The drawing under review shows one solid part. Ordinate dimensions are in mm from its lowest x, y, z. A direction names the side the tool comes from. Round coordinates to 2 decimals unless told otherwise and drop trailing zeros. Order: outer loops, then holes, each group sorted by start corner. A loop starts at its lowest first (then second) coordinate and runs counter-clockwise, first axis right, second up.
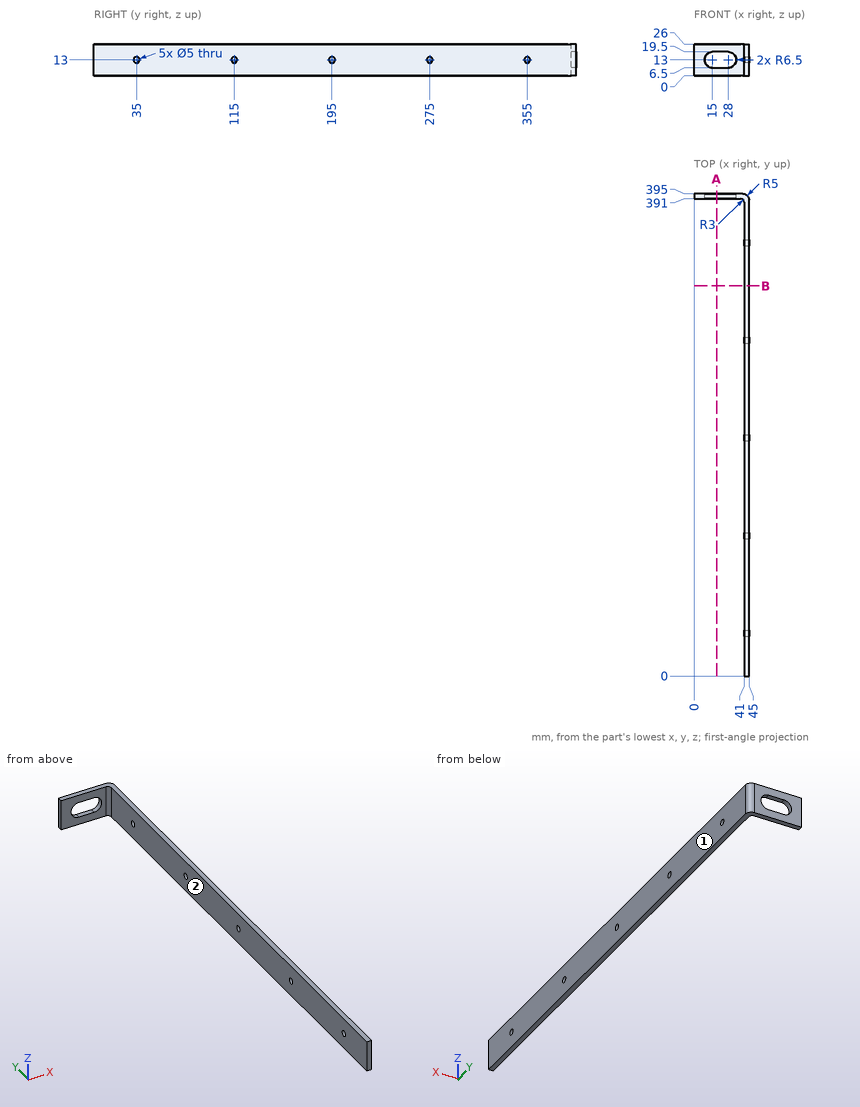
Q1. Clearance check with flat-ended pins moving along their axes: pin 1 (6.5 mm diameter, centred on y = 355, z = 13, fed in from -X); pin 2 (10 mm diameter, centred on x = 5.5, z = 19, fed in from -Y). State where each tip first meets the part, or that it passes through.
Q2. Take a section at A-A, the plane x = 18.5. State the section outline as (y, z) points, plus the area to 3 significant figures.
Q3. Wall thickness on line 1 (Z direction, x = 42.75, y = 195); line 2 (Y direction, x = 42.45, z = 13); line 3 (Y direction, x = 41.9, z = 13): over which ranges is each line inside the solid? List them lowest first.
Q4. Take a section at B-B, the plane y = 319.5. State the section outline as (x, z) points, plus the area to 3 significant figures.
Q5. Tool access review of the marked faces 1 and 2: name each direction out of +Z, -Z, +X, -X, +Y, -Y from which nothing blocks a thin tool from reaching the whole face with its end or side.
Working result:
1. pin 1: stops at x = 41
1. pin 2: stops at y = 391
2. outline: (391, 0) - (395, 0) - (395, 6.5) - (391, 6.5) - close; (391, 19.5) - (395, 19.5) - (395, 26) - (391, 26) - close
2. area: 52.0 mm2
3. line 1: z = 0 to 10.5, 15.5 to 26
3. line 2: y = 0 to 32.5, 37.5 to 112.5, 117.5 to 192.5, 197.5 to 272.5, 277.5 to 352.5, 357.5 to 394.36
3. line 3: y = 0 to 32.5, 37.5 to 112.5, 117.5 to 192.5, 197.5 to 272.5, 277.5 to 352.5, 357.5 to 394.62
4. outline: (41, 0) - (45, 0) - (45, 26) - (41, 26) - close
4. area: 104 mm2
5. face 1: +Z, -Z, +X, +Y, -Y
5. face 2: +Z, -Z, -X, -Y
